Geometry check sheet. Reference: the model listing, model coordinates, mm. Coordinates: 2 decimals unless noted, no trailing zeros. Write each loop counter-clockwise with the first axis right and the second up, starting at its lowest first coordinate (ties: lowest second). Pieces come first, ordered by that corner, then holes. Notation, with made-up numbers: (62.5, 67.5) -> (118.5, 67.5) arc R26 ccw to (118.5, 84.5) -> close; hole circle Ø2 at (-28, 60). An arc over 180 degrees is marked (long way). Answer as CSV lines item,"result".
```python
from build123d import *

# Parameters (mm, degrees)
MODEL_R                 = 4.5
MODEL_R_2               = 1.5
SALIENTE_EXTRUIR1_DEPTH = 3


with BuildPart() as part:
    # Model → Saliente-Extruir1 (new body)
    with BuildSketch(Plane.XY):
        with BuildLine():
            Line((196.727054575, 226.678720063), (178.727054575, 226.678720063))
            ThreePointArc((178.727054575, 226.678720063), (175.545074059, 225.360700578), (174.227054575, 222.178720063))
            Line((174.227054575, 222.178720063), (174.227054575, 213.178720063))
            Line((174.227054575, 213.178720063), (174.227054575, 199.678720063))
            ThreePointArc((174.227054575, 199.678720063), (174.569596678, 197.956644617), (175.545074059, 196.496739548))
            Line((175.545074059, 196.496739548), (184.545074059, 187.496739548))
            ThreePointArc((184.545074059, 187.496739548), (187.727054575, 186.178720063), (190.90903509, 187.496739548))
            Line((190.90903509, 187.496739548), (199.90903509, 196.496739548))
            ThreePointArc((199.90903509, 196.496739548), (200.884512471, 197.956644617), (201.227054575, 199.678720063))
            Line((201.227054575, 199.678720063), (201.227054575, 222.178720063))
            ThreePointArc((201.227054575, 222.178720063), (199.90903509, 225.360700578), (196.727054575, 226.678720063))
        make_face()
        with Locations((187.727054575, 195.178720063)):
            Circle(MODEL_R, mode=Mode.SUBTRACT)
        with Locations((187.727054575, 204.178720063)):
            Circle(MODEL_R_2, mode=Mode.SUBTRACT)
        with Locations((178.727054575, 204.178720063)):
            Circle(MODEL_R_2, mode=Mode.SUBTRACT)
        with Locations((187.727054575, 213.178720063)):
            Circle(MODEL_R_2, mode=Mode.SUBTRACT)
        with Locations((178.727054575, 213.178720063)):
            Circle(MODEL_R_2, mode=Mode.SUBTRACT)
        with Locations((196.727054575, 213.178720063)):
            Circle(MODEL_R_2, mode=Mode.SUBTRACT)
        with Locations((196.727054575, 204.178720063)):
            Circle(MODEL_R_2, mode=Mode.SUBTRACT)
        with Locations((187.727054575, 222.178720063)):
            Circle(MODEL_R_2, mode=Mode.SUBTRACT)
        with Locations((178.727054575, 222.178720063)):
            Circle(MODEL_R_2, mode=Mode.SUBTRACT)
        with Locations((196.727054575, 222.178720063)):
            Circle(MODEL_R_2, mode=Mode.SUBTRACT)
    extrude(amount=SALIENTE_EXTRUIR1_DEPTH)


solid = part.part
```
Item 1: Cross-section at D-D, the plane y = 189. Record the cut outline in (x, z).
Responses:
outline,"(183.04, 0) -> (192.41, 0) -> (192.41, 3) -> (183.04, 3) -> close"
Item 2: Depth check by flat-ended pin: pin 1 Ø4 at (x, y) = (196.73, 213.18) entering from -Z. Enter the tip coordinate at first touch or a pass-through.
Responses:
pin 1,"stops at z = 0"
Item 3: Release check for a two-part mould opening along X. For faces 1 (the cylindrical face through (188.533, 214.444, 1.479)), 2 (the cylindrical face through (174.56, 197.98, 1.48)), 3 (the cylindrical face through (199.94, 225.33, 1.48)) record: +X half, -X half, draft (parallel to the pull), parting line (faces both ways), or undercut.
Responses:
face 1,"undercut"
face 2,"-X half"
face 3,"+X half"
Item 4: Cross-section at C-C, the plane x = 186.75. Record the cut outline in (y, z).
Responses:
outline,"(186.29, 0) -> (190.79, 0) -> (190.79, 3) -> (186.29, 3) -> close; (199.57, 0) -> (203.04, 0) -> (203.04, 3) -> (199.57, 3) -> close; (205.32, 0) -> (212.04, 0) -> (212.04, 3) -> (205.32, 3) -> close; (214.32, 0) -> (221.04, 0) -> (221.04, 3) -> (214.32, 3) -> close; (223.32, 0) -> (226.68, 0) -> (226.68, 3) -> (223.32, 3) -> close"
Item 5: Thickness scan on probe 1 along Y at (x, z) = (187.75, 2); probe 2 along X at (y, z) = (205, 1.85); probe 3 along Y at (x, z) = (188.75, 2.7). Record the ranges inside material, lowest first.
Responses:
probe 1,"y = 186.18 to 190.68, 199.68 to 202.68, 205.68 to 211.68, 214.68 to 220.68, 223.68 to 226.68"
probe 2,"x = 174.23 to 177.47, 179.98 to 186.47, 188.98 to 195.47, 197.98 to 201.23"
probe 3,"y = 186.3 to 190.8, 199.56 to 203.08, 205.28 to 212.08, 214.28 to 221.08, 223.28 to 226.68"
Item 6: Cross-section at B-B, the plane z = 0.9. Count the separate pieces of the cut face and the enclosed holes in it, plus the area to 3 significant figures.
Responses:
separate pieces,"1"
enclosed holes,"10"
area,"820 mm2"
Item 7: Cross-section at A-A, the plane y = 197.5. Record the cut outline in (x, z).
Responses:
outline,"(174.79, 0) -> (183.87, 0) -> (183.87, 3) -> (174.79, 3) -> close; (191.58, 0) -> (200.66, 0) -> (200.66, 3) -> (191.58, 3) -> close"
